Here's how the part is built. I have some questions about the finished solid (model axes, mm). A direction names the side the tool comes from. Give positions to 0.01 mm unless a question says otherwise; leave off trailing zeros. Write each loop counter-clockwise with the first axis right and the second up, starting at its lowest first coordinate (ties: lowest second). Pieces come first, ordered by that corner, then holes. Notation, with made-up numbers: (10, -29.5) - (33, -29.5) arc R28 cw to (33, 8.5) - close; hole circle Ø1 at (-13, 33). An arc over 180 degrees is marked (long way). Use a Markdown table: item, result.
```python
from build123d import *

# Parameters (mm, degrees)
BOSS_EXTRUDE1_DEPTH      = 10
BOSS_EXTRUDE1_DEPTH_BACK = 10
SKETCH1_R                = 7.5
SKETCH3_R                = 7.5
BOSS_EXTRUDE2_DEPTH      = 20
SKETCH4_R                = 5.005
CUT_EXTRUDE2_DEPTH       = 23
SKETCH5_R                = 5.005
CUT_EXTRUDE3_DEPTH       = 9


with BuildPart() as part:
    # Sketch1 → Boss-Extrude1 (new, two sides: drawn at the far end of the back side and taken through both)
    with BuildSketch(Plane.XY.offset(-BOSS_EXTRUDE1_DEPTH_BACK)):
        Circle(SKETCH1_R)
    extrude(amount=BOSS_EXTRUDE1_DEPTH + BOSS_EXTRUDE1_DEPTH_BACK)

    # Sketch3 → Boss-Extrude2 (add)
    with BuildSketch(Plane(origin=(0, 20, 0), x_dir=(1, 0, 0), z_dir=(0, 1, 0))):
        with Locations(Location((0, 0, 0), (0, 0, 270))):
            Circle(SKETCH3_R)
    extrude(amount=-BOSS_EXTRUDE2_DEPTH)

    # Sketch4 → Cut-Extrude2 (cut)
    with BuildSketch(Plane.XY.offset(10)):
        Circle(SKETCH4_R)
    extrude(amount=-CUT_EXTRUDE2_DEPTH, mode=Mode.SUBTRACT)

    # Sketch5 → Cut-Extrude3 (cut)
    with BuildSketch(Plane(origin=(0, 20, 0), x_dir=(1, 0, 0), z_dir=(0, 1, 0))):
        with Locations(Location((0, 0, 0), (0, 0, 270))):
            Circle(SKETCH5_R)
    extrude(amount=-CUT_EXTRUDE3_DEPTH, mode=Mode.SUBTRACT)


solid = part.part
```
Item 1: If we section it at C-C, the plane y = -3: Write out the boundary of the cut face in (x, z), plus the area to 3 significant figures.
Values:
| item | result |
|---|---|
| outline | (-6.87, -10) - (-4.01, -10) - (-4.01, 10) - (-6.87, 10) - close; (4.01, -10) - (6.87, -10) - (6.87, 10) - (4.01, 10) - close |
| area | 115 mm2 |
Item 2: Will these pins go through, and if not, where does the flat tip stop? pin 1 Ø2 at (y, z) = (-4.5, -7.5) entering from -X; pin 2 Ø4 at (y, z) = (-4.5, -4) entering from +X; pin 3 Ø8 at (x, z) = (5, 6) entering from +Y; pin 4 Ø1 at (y, z) = (1, 1) entering from +X.
Values:
| item | result |
|---|---|
| pin 1 | stops at x = -6.63 |
| pin 2 | stops at x = 7.07 |
| pin 3 | stops at y = 20 |
| pin 4 | stops at x = 7.48 |
Item 3: I need wall thicknesses on line 1 along X through (y, z) = (15.25, 0) (3 decimals); line 2 along Y through (x, z) = (0, -3.25) (3 decimals); line 3 along X through (y, z) = (6, 0.25). Which ranges of each line are inside material? Lowest first, please. Write a range as [from, to].
Values:
| item | result |
|---|---|
| line 1 | x = [-7.5, -5.005], [5.005, 7.5] |
| line 2 | y = [-7.5, -5.005], [5.005, 11] |
| line 3 | x = [-7.5, 7.5] |
Item 4: Thinking about a two-plate mould opening in X: for faces 3 (the cylindrical face through (-3.05, 15.56, -3.97)), 4 (the flat face through (-5, 20, 2)), 5 (the cylindrical face through (-1.63, -7.32, -0.14)), which applies, +X half, -X half, draft (parallel to the pull), parting line (faces both ways), or undercut?
Values:
| item | result |
|---|---|
| face 3 | undercut |
| face 4 | draft |
| face 5 | parting line |
Item 5: If we section it at D-D, the plane x = 2.75: Write out the boundary of the cut face in (y, z).
Values:
| item | result |
|---|---|
| outline | (-6.98, -10) - (-4.18, -10) - (-4.18, 10) - (-6.98, 10) - close; (4.18, -10) - (6.98, -10) - (6.98, -6.98) - (20, -6.98) - (20, -4.18) - (11, -4.18) - (11, 4.18) - (20, 4.18) - (20, 6.98) - (6.98, 6.98) - (6.98, 10) - (4.18, 10) - close |
Item 6: If we section it at B-B, the plane z = 0: Write out the boundary of the cut face in (x, y) (3 decimals).
Values:
| item | result |
|---|---|
| outline | (-7.5, 0) arc R7.5 ccw to (7.5, 0) - (7.5, 20) - (5.005, 20) - (5.005, 11) - (-5.005, 11) - (-5.005, 20) - (-7.5, 20) - close; hole circle Ø10.01 at (0, 0) |
Item 7: For faces 1 (the flat face through (0, 11, 0)), 2 (the cylindrical face through (-3.97, -3.05, 0.14)), which set-ups out of +Z, -Z, +X, -X, +Y, -Y let a thin tool reach every point of the face, with its end or its side?
Values:
| item | result |
|---|---|
| face 1 | +Y |
| face 2 | +Z, -Z |
Item 8: If we section it at A-A, the plane x = 0: Write out the boundary of the cut face in (y, z) (3 decimals).
Values:
| item | result |
|---|---|
| outline | (-7.5, -10) - (-5.005, -10) - (-5.005, 10) - (-7.5, 10) - close; (5.005, -10) - (7.5, -10) - (7.5, -7.5) - (20, -7.5) - (20, -5.005) - (11, -5.005) - (11, 5.005) - (20, 5.005) - (20, 7.5) - (7.5, 7.5) - (7.5, 10) - (5.005, 10) - close |
